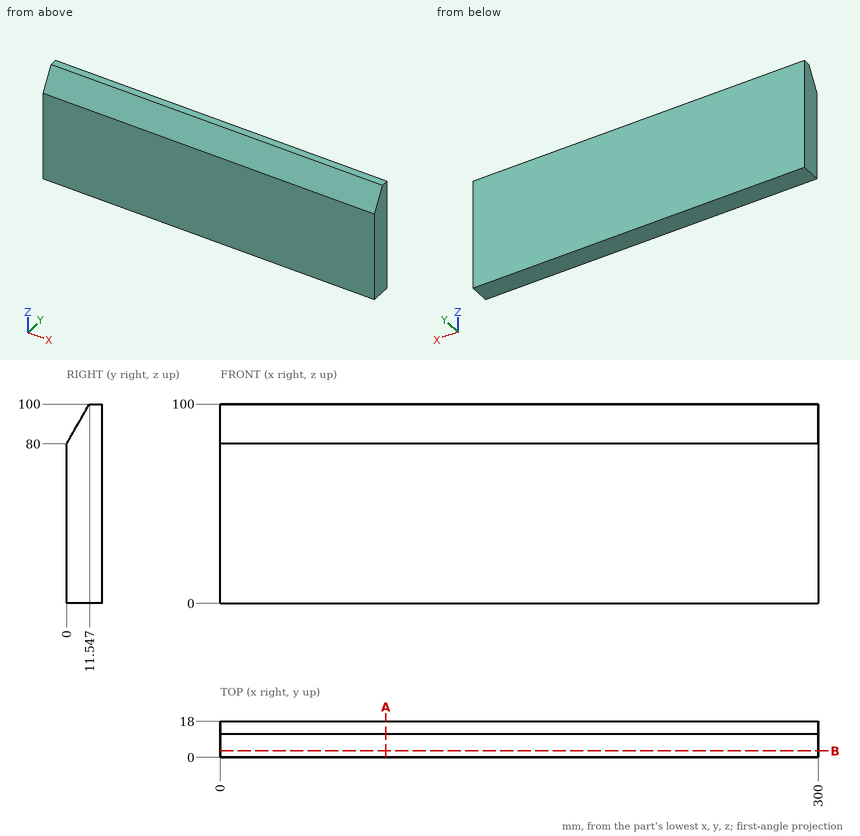
For this review, use the dimensioned drawing (mm, ordinates from the lowest corner) and the shaded views. Give positions to 0.01 mm unless a question says otherwise; leave off trailing zeros. Loops run counter-clockwise (first coordinate to the right, second up) from the corner with the lowest first, then second, coordinate; pieces in that order, holes last.
Item 1: Take a section at A-A, the plane x = 83. State the section outline as (y, z) points.
Item 2: Take a section at B-B, the plane y = 3.25. State the section outline as (x, z) points.
Item 3: For line 1 along Z through (x, y) = (211, 11.25); line 2 along Y through (x, z) = (150.5, 80.5); line 3 along Z through (x, y) = (208, 2.5), list the stretches that pass through material, from the lowest coordinate up.
Item 4: Insertion check: pin 1 (3 mm diameter, centred on x = 131, y = 14.5, fed in from -Z). The pin has a flat end and moves straight along its axis. Give the tip position at first contact, or say it passes through.
Calculated:
1. outline: (0, 0) - (18, 0) - (18, 100) - (11.55, 100) - (0, 80) - close
2. outline: (0, 0) - (300, 0) - (300, 85.63) - (0, 85.63) - close
3. line 1: z = 0 to 99.49
3. line 2: y = 0.29 to 18
3. line 3: z = 0 to 84.33
4. pin 1: stops at z = 0
